```python
from build123d import *

# Parameters (mm, degrees)
F0_W     = 60
F0_H     = 34
F1_DEPTH = 5
F2_R     = 3
F3_DEPTH = 2.5
F4_R     = 1.85
F5_DEPTH = 2.501
F6_R     = 1.4732
F7_DEPTH = 3.175


with BuildPart() as f1:
    # F0 (on Top) → F1 (new body)
    with BuildSketch(Plane.XY):
        Rectangle(F0_W, F0_H)
    extrude(amount=F1_DEPTH)

    # F2 (on face) → F3 (cut)
    with BuildSketch(Plane.XY.offset(5)):
        with Locations((0, 10)):
            Circle(F2_R)
        with Locations((0, -10)):
            Circle(F2_R)
    extrude(amount=-F3_DEPTH, mode=Mode.SUBTRACT)

    # F4 (on face) → F5 (cut, through all)
    with BuildSketch(Plane.XY.offset(2.5)):
        with Locations((0, 10)):
            Circle(F4_R)
        with Locations((0, -10)):
            Circle(F4_R)
    extrude(amount=-F5_DEPTH, mode=Mode.SUBTRACT)

    # F6 (on face) → F7 (join)
    with BuildSketch(Plane.XY.offset(5)):
        with Locations((-15.875, 10.65)):
            Circle(F6_R)
        with Locations((15.875, 10.65)):
            Circle(F6_R)
    extrude(amount=F7_DEPTH)


solid = f1.part
```
Source: CAD feature listing. Evaluate the final solid. Frame: model axes, mm. A direction names the side the tool comes from. Round coordinates to 2 decimals unless told otherwise and drop trailing zeros. Loops run counter-clockwise (first coordinate to the right, second up) from the corner with the lowest first, then second, coordinate; pieces in that order, holes last. Notation, with made-up numbers: M 78.5,37.5 L 88.5,37.5 A27 cw 88.5,62.5 Z; hole C 7.5,-12 d1. An arc over 180 degrees is marked long. Put each result on its own line as item: value.
(1) Section D-D, the plane x = -6. Return loops of the section in (y, z).
Solutions:
outline: M -17,0 L 17,0 L 17,5 L -17,5 Z
(2) Section C-C, the plane y = 10. Return loops of the section in (x, z) (3 decimals), and give its area (3 significant figures).
Solutions:
outline: M -30,0 L -1.85,0 L -1.85,2.5 L -3,2.5 L -3,5 L -14.553,5 L -14.553,8.175 L -17.197,8.175 L -17.197,5 L -30,5 Z; M 1.85,0 L 30,0 L 30,5 L 17.197,5 L 17.197,8.175 L 14.553,8.175 L 14.553,5 L 3,5 L 3,2.5 L 1.85,2.5 Z
area: 293 mm²
(3) Access query for faces 1 (the face through (0, 17, 2)), 2 (the face through (-14.514, 10.086, 6.565)). Directions: +Z, -Z, +X, -X, +Y, -Y. A direction counts if a zero-diameter tool reaches every point of the face in a straight line with its end or side. Return the directions, or none.
Solutions:
face 1: +Z, -Z, +X, -X, +Y
face 2: +Z
(4) Ray query, line 1 (Y direction, x = 0, z = 1.35); line 2 (Y direction, x = 0, z = 2.75); line 3 (Z direction, x = 3, y = 7). Return the intervals inside material, ascending. Write a range as [from, to].
Solutions:
line 1: [-17, -11.85], [-8.15, 8.15], [11.85, 17]
line 2: [-17, -13], [-7, 7], [13, 17]
line 3: [0, 5]
(5) Section B-B, the plane x = 0. Return loops of the section in (y, z).
Solutions:
outline: M -17,0 L -11.85,0 L -11.85,2.5 L -13,2.5 L -13,5 L -17,5 Z; M -8.15,0 L 8.15,0 L 8.15,2.5 L 7,2.5 L 7,5 L -7,5 L -7,2.5 L -8.15,2.5 Z; M 11.85,0 L 17,0 L 17,5 L 13,5 L 13,2.5 L 11.85,2.5 Z
(6) Pull-direction query (Y, two-part tool) for faces 3 (the face through (30, 0, 2)), 4 (the face through (17.236, 10.086, 6.565)), 5 (the face through (0, 8, 2.5)); classes: released by +Y, released by -Y, zero draft, split by the parting line, or undercut.
Solutions:
face 3: zero draft
face 4: split by the parting line
face 5: undercut
(7) Section A-A, the plane y = -10. Return loops of the section in (x, z), and give its area (3 significant figures).
Solutions:
outline: M -30,0 L -1.85,0 L -1.85,2.5 L -3,2.5 L -3,5 L -30,5 Z; M 1.85,0 L 30,0 L 30,5 L 3,5 L 3,2.5 L 1.85,2.5 Z
area: 276 mm²
(8) First-contact query: pin 1 (8 mm diameter, centred on x = 0, y = 10, fed in from -Z); pin 2 (4 mm diameter, centred on x = 5.5, y = 12.5, fed in from +Z); pin 3 (5 mm diameter, centred on x = 0, y = -10, fed in from +Z). Flat tips, straight axial feed; report the tip coordinate or a pass-through.
Solutions:
pin 1: z = 0
pin 2: z = 5
pin 3: z = 2.5
